Autodesk Inventor part; units mm, degrees
ref_plane "YZ Plane" through (0, 0, 0) normal (1, 0, 0) x (0, 1, 0)
ref_plane "XZ Plane" through (0, 0, 0) normal (0, 1, 0) x (-1, 0, 0)
ref_plane "XY Plane" through (0, 0, 0) normal (0, 0, 1) x (1, 0, 0)
sketch "axes" plane through (0, 0, 0) normal (0, 0, 1) x (1, 0, 0)
  point P0 (0, 0)
  point P1 (-40, 0)
  point P2 (0, 0)
  dimension "d0" = 40
sketch "tendon anchors" plane through (0, 0, 0) normal (0, 0, 1) x (1, 0, 0)
  line L0 (-8.2564, 0) -> (0, 0) construction
  line L1 (0, 0) -> (-7.5, -7.5) construction
  line L2 (-32.0254, 0) -> (-40, 0) construction
  line L3 (-40, 0) -> (-30.5, -5.5) construction
  dimension "d136" = 7.5
  dimension "d137" = 7.5
  dimension "d138" = 5.5
  dimension "d139" = 9.5
sketch "Sketch3" plane through (0, 0, 0) normal (0, 0, 1) x (1, 0, 0)
  line L0 (-48, 9) -> (8, 9)
  line L1 (8, 9) -> (8, -9)
  line L2 (8, -9) -> (-48, -9)
  line L3 (-48, -9) -> (-48, 9)
  point P0 (0, 0)
  point P1 (8, 0)
  point P2 (-40, 0)
  dimension "d1" = 18
  dimension "d2" = 8
  dimension "d3" = 8
extrude "base plate" add sketch "Sketch3" along normal blind 2
sketch "Sketch4" plane through (0, 0, 2) normal (0, 0, 1) x (1, 0, 0)
  line L0 (8, 9) -> (-48, 9)
  line L1 (-48, 9) -> (-48, -9)
  line L2 (-48, -9) -> (8, -9)
  line L3 (8, -9) -> (8, 9)
  line L4 (-31.5, 9) -> (-8, 9)
  line L5 (-8, 9) -> (-8, 5.4)
  line L6 (-8, 5.4) -> (-31.5, 5.4)
  line L7 (-31.5, 5.4) -> (-31.5, 9)
  line L8 (-30.5, -9) -> (-7.5, -9)
  line L9 (-7.5, -9) -> (-7.5, -4)
  line L10 (-7.5, -4) -> (-30.5, -4)
  line L11 (-30.5, -4) -> (-30.5, -9)
  point P0 (0, 0)
  point P1 (-30.5, -5.5)
  point P2 (-7.5, -7.5)
  dimension "d6" = 5
  dimension "d7" = 3.6
  dimension "d8" = 16.5
  dimension "d9" = 16
extrude "walls" add sketch "Sketch4" along normal blind 4.5 contours L5 L6 L7 L0 | L2 L11 L10 L9
sketch "Sketch5" plane through (0, 0, 2) normal (0, 0, 1) x (1, 0, 0)
  point P0 (0, 0)
  point P1 (-40, 0)
  point P2 (0, 0)
hole "joint bearings" at (-40, 0, 2) direction (0, 0, -1) diameter 3.5 end through all counterbore diameter 5 counterbore depth 1.5
fillet "front top" radius 5 1 edges at (-48, 9, 1)
fillet "front bottom" radius 8 1 edges at (-48, -9, 1)
sketch "Sketch7" plane through (0, 0, 2) normal (0, 0, 1) x (1, 0, 0)
  circle A0 centre (-40, 0) radius 4
  line L0 (-31.5, 9) -> (-43, 9)
  arc A1 (-43, 9) -> (-48, 4) centre (-43, 4) ccw
  line L1 (-31.5, 5.4) -> (-31.5, 9)
  line L2 (-43.3321, 8.989) -> (-37.1716, 2.8284)
  line L3 (-40, 0) -> (-52.831, 0) construction
  line L4 (-31.5, 5.4) -> (-39.7431, 5.4)
  point P0 (0, 0)
  dimension "d33" = 8
  dimension "d34" = 45
extrude "extension endstop" add sketch "Sketch7" along normal blind 2 contours L2 A1 L0 L1 L4
sketch "Sketch8" plane through (0, 0, 2) normal (0, 0, 1) x (1, 0, 0)
  point P0 (0, 0)
  point P1 (-40, 0)
  point P2 (-19.5, 2.5)
  point P3 (-19.5, 2.5)
  point P4 (-19.5, -1.5)
  dimension "d41" = 20.5
  dimension "d73" = 2.5
  dimension "d127" = 1.5
hole "spring pin" at (-19.5, 2.5, 2) at (-19.5, -1.5, 2) direction (0, 0, -1) diameter 1.5 end through all
sketch "Sketch10" plane through (0, 0, 2) normal (0, 0, 1) x (1, 0, 0)
  line L0 (-9, -9) -> (8, -9)
  line L1 (8, -9) -> (8, 9)
  line L2 (8, 9) -> (-9, 9)
  line L3 (-9, 9) -> (-9, -9)
  point P0 (0, 0)
  point P1 (-8, 9)
  dimension "d126" = 17
extrude "Extrusion4" add sketch "Sketch10" along normal blind 1
sketch "Sketch11" plane through (0, 0, 0) normal (0, 0, -1) x (-1, 0, 0)
  circle A0 centre (0, 0) radius 9
  line L0 (0, 9) -> (-9, 9)
  line L1 (-9, 9) -> (-9, -9)
  line L2 (-9, -9) -> (9, -9)
  line L3 (9, -9) -> (9, 0)
  dimension "d57" = 18
extrude "Extrusion5" cut sketch "Sketch11" against normal blind 1.5
fillet "Fillet5" radius 1 2 edges at (0, 9, 0.75) (-9, -9, 0.75)
fillet "Fillet6" radius 5 1 edges at (8, 9, 2.25)
fillet "Fillet7" radius 9 1 edges at (8, -9, 2.25)
sketch "Sketch12" plane through (0, 0, 3) normal (0, 0, 1) x (1, 0, 0)
  circle A0 centre (0, 0) radius 1.75
  line L0 (-0.75, -1.5811) -> (-0.75, 1.5811)
  dimension "d63" = 3.5
  dimension "d140" = 0.75
extrude "Extrusion6" cut sketch "Sketch12" against normal blind 1 contours A0 L0 picked at (0.0833, 0)
sketch "Sketch18" plane through (0, 0, 6.5) normal (0, 0, 1) x (1, 0, 0)
  line L0 (-31.5, 9) -> (-31.5, 5.4)
  line L1 (-31.5, 5.4) -> (-8, 5.4)
  line L2 (-8, 5.4) -> (-8, 9)
  line L3 (-8, 9) -> (-31.5, 9)
  line L4 (-30.5, -9) -> (-7.5, -9)
  line L5 (-7.5, -9) -> (-7.5, -4)
  line L6 (-7.5, -4) -> (-30.5, -4)
  line L7 (-30.5, -4) -> (-30.5, -9)
  circle A0 centre (-19.5, 2.5) radius 0.75
  line L8 (-21.5, 5.4) -> (-17.5, 5.4)
  line L9 (-17.5, 5.4) -> (-17.5, -4)
  line L10 (-17.5, -4) -> (-21.5, -4)
  line L11 (-21.5, -4) -> (-21.5, 5.4)
  line L12 (-19.5, 2.5) -> (-19.5, -2.026) construction
  point P0 (0, 0)
  dimension "d105" = 4
extrude "Extrusion8" add sketch "Sketch18" along normal blind 1.5 contours L3 L2 L1 L0 | L1 L9 L6 L11 | L6 L5 L4 L7 | A0
sketch "Sketch19" plane through (0, 0, 6.5) normal (0, 0, -1) x (-1, 0, 0)
  circle A0 centre (19.5, 2.5) radius 0.75
  circle A1 centre (19.5, -1.5) radius 0.75
  point P0 (0, 0)
hole "spring pins support" at (-19.5, 2.5, 6.5) at (-19.5, -1.5, 6.5) direction (0, 0, 1) diameter 1 end through all counterbore diameter 1.5 counterbore depth 1.25
sketch "Sketch14" plane through (0, 0, 3) normal (0, 0, 1) x (1, 0, 0)
  line L0 (-0.75, -1.5811) -> (-0.75, 1.5811)
  arc A0 (-0.75, -1) -> (-0.75, 1) centre (0, 0) ccw
  dimension "d133" = 2.5
extrude "Extrusion11" cut sketch "Sketch14" against normal through all
sketch "Sketch17" plane through (0, 0, 8) normal (0, 0, 1) x (1, 0, 0)
  point P0 (0, 0)
  point P1 (-26, -7)
  point P2 (-13, -7)
  point P3 (-29.5, 7)
  point P4 (-10.5, 7)
  point P5 (-40, 0)
  point P6 (0, 0)
  point P7 (-40, 0)
  point P8 (0, 0)
  dimension "d92" = 7
  dimension "d93" = 7
  dimension "d94" = 10.5
  dimension "d95" = 10.5
  dimension "d96" = 14
  dimension "d97" = 13
hole "mounting" at (-29.5, 7, 8) at (-10.5, 7, 8) at (-26, -7, 8) at (-13, -7, 8) direction (0, 0, -1) diameter 1.6 depth 6 tip angle 118
sketch "Sketch20" plane through (-48, 4, 0) normal (-1, 0, 0) x (0, 0, 1)
  line L0 (3, 5) -> (20, 5)
  line L1 (20, 5) -> (20, -13)
  line L2 (20, -13) -> (3, -13)
  line L3 (0, -10) -> (0, 2)
  arc A0 (3, 5) -> (0, 2) centre (3, 2) ccw
  arc A1 (0, -10) -> (3, -13) centre (3, -10) ccw
  point P0 (0, -4)
  point P1 (0, 5)
  point P2 (0, -13)
  point P3 (0, -13)
  dimension "d115" = 20
  dimension "d116" = 3
extrude "side fillet" cut sketch "Sketch20" against normal through all keep common part
fillet "Fillet8" radius 1 5 edges at (-44.0048, -7.9255, 0.6994) (-48, 1.5, 0) (-47.8945, 5.0215, 0) (-46.0631, 7.9519, 0.7218) (-47.5485, -3.6495, 0)
sketch "Sketch21" plane through (-43, 9, 4) normal (0, 1, 0) x (1, 0, 0)
  line L0 (11.5, 0) -> (0, 0)
  line L1 (11.5, 0) -> (11.5, -4)
  line L2 (10, -4) -> (10, -4) construction
  line L3 (11.15, -4) -> (11.15, -4)
  line L4 (8.85, -4) -> (8.85, -4)
  arc A0 (8.85, -4) -> (11.15, -4) centre (10, -4) ccw
  arc A1 (11.15, -4) -> (8.85, -4) centre (10, -4) ccw
  line L5 (8.85, -4) -> (7.85, -4)
  line L6 (7.85, -4) -> (7.85, 0)
  line L7 (11.15, -4) -> (11.5, -4)
  point P0 (43, 4)
  point P1 (10, -3.75)
  point P2 (3, 4)
  dimension "d120" = 2.3
  dimension "d121" = 7
  dimension "d122" = 0
  dimension "d123" = 1
extrude "cable clip" add sketch "Sketch21" against normal blind 3 contours L1 L7 A1 L5 L6 L0
chamfer "Chamfer1" distance 1 angle 45 3 edges at (-9, 0.7, 2) (-24.3716, 5.4, 2) (-19.75, -4, 2)
fillet "Fillet9" radius 1 4 edges at (-21.5, 5.4, 7.25) (-17.5, 5.4, 7.25) (-17.5, -4, 7.25) (-21.5, -4, 7.25)
fillet "Fillet10" radius 1 4 edges at (-22, -4, 6.5) (-17, -4, 6.5) (-17, 5.4, 6.5) (-22, 5.4, 6.5)
equation "\"MCP_PIP_length\" = F4_MCP_PIP_length"
equation "\"PIP_spring_length\" = F4_PIP_spring_length"
properties part number "phalanx 1 R F4"
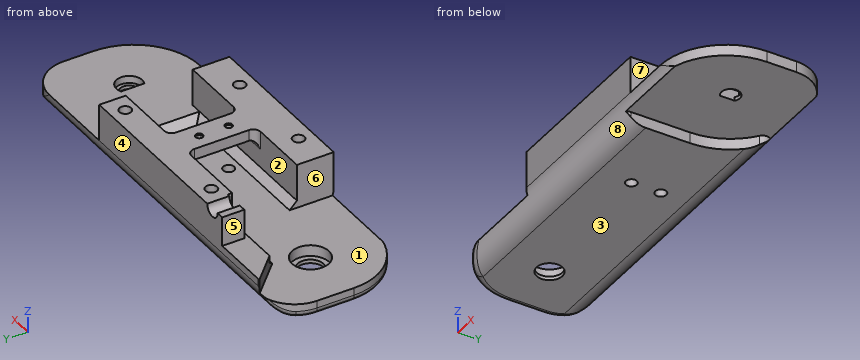
Design review of the part built by this model. Coordinates are the model's own, in mm. Face numbers are marked on the shaded views. A direction names the side the tool comes from. Round coordinates to 2 decimals unless told otherwise and drop trailing zeros. Write each loop counter-clockwise with the first axis right and the second up, starting at its lowest first coordinate (ties: lowest second). Pieces come first, ordered by that corner, then holes. Notation, with made-up numbers: (58.25, -4) -> (100.25, -4) arc R5 cw to (100.25, 2) -> close; hole circle Ø11 at (77, -4.75). An arc over 180 degrees is marked (long way). Write item = value, one per line. Start each with the question number.
1) Clearance check with flat-ended pins moving along their axes: pin 1 (1.5 mm diameter, centred on x = -13.5, y = 3, fed in from +Z); pin 2 (1.5 mm diameter, centred on x = -40.5, y = 1, fed in from +Z); pin 3 (1.4 mm diameter, centred on x = -26, y = -7, fed in from +Z). State where each tip first meets the part, or that it passes through.
2) Take a section at B-B, the plane x = 0. State the section outline as (y, z) points.
3) Wall thickness on probe 1 along Y at (x, z) = (-29.5, 6.7); probe 2 along X at (y, z) = (2.5, 6.9); probe 3 along Y at (x, z) = (-11, 5.25): over which ranges is each line inside the solid? List them lowest first. Write a range as from..to.
4) Tool access review of the marked faces 5, 6, 7 and 8: name each direction out of +Z, -Z, +X, -X, +Y, -Y from which nothing blocks a thin tool from reaching the whole face with its end or side.
5) Take a section at D-D, the plane x = -32.5. State the section outline as (y, z) points.
6) Take a section at A-A, the plane z = 4.75. State the section outline as (x, y) points, plus the area to 3 significant figures.
7) Mouldability with a two-part tool opening along Y and no side actions: class the marked faces 1, 2, 3 and 4 as +Y half, -Y half, draft (parallel to the pull), parting line (faces both ways), or undercut.
8) Take a section at C-C, the plane x = -19.5. Count the separate pieces of the cut face and the enclosed holes in it, plus the area to 3 significant figures.
Results list:
q1.pin_1 = 2
q1.pin_2 = 0.5
q1.pin_3 = 1.94
q2.outline = (-8.94, 2.42) arc R3 ccw to (-8.6, 1.5) -> (-1.25, 1.5) -> (-1.25, 2) -> (-1.75, 2) -> (-1.75, 3) -> (-8.94, 3) -> close; (1.25, 1.5) -> (8.6, 1.5) arc R3 ccw to (9, 3) -> (1.75, 3) -> (1.75, 2) -> (1.25, 2) -> close
q3.probe_1 = -9..-4, 5.4..6.2, 7.8..9
q3.probe_2 = -21.5..-20.25, -18.75..-17.5
q3.probe_3 = -9..-4, 5.4..6.38, 7.62..9
q4.face_5 = +Z, -X, +Y, -Y
q4.face_6 = +Z, -X, -Y
q4.face_7 = +Z, +X, +Y, -Y
q4.face_8 = -Z, +X, -X, -Y
q5.outline = (-8.83, 2) arc R3 ccw to (-6, 0) -> (6, 0) arc R3 ccw to (9, 3) -> (9, 6.96) -> (6, 6.96) -> (6, 4) -> (5.4, 4) -> (5.4, 3) -> (4.4, 2) -> close
q6.outline = (-35.15, 6) -> (-31.5, 6) -> (-31.5, 5.4) -> (-8, 5.4) -> (-8, 9) -> (-35.15, 9) -> close; (-30.5, -9) -> (-7.5, -9) -> (-7.5, -4) -> (-30.5, -4) -> close; hole circle Ø1.6 at (-29.5, 7); hole circle Ø1.6 at (-26, -7); hole circle Ø1.6 at (-13, -7); hole circle Ø1.6 at (-10.5, 7)
q6.area = 203 mm²
q7.face_1 = undercut
q7.face_2 = undercut
q7.face_3 = draft
q7.face_4 = +Y half
q8.separate_pieces = 4
q8.enclosed_holes = 0
q8.area = 89.0 mm²
